CAD build for the part. Positions are in the model's coordinates, mm. Face numbers are marked on the shaded views. A direction names the side the tool comes from. Round coordinates to 2 decimals unless told otherwise and drop trailing zeros. Write each loop counter-clockwise with the first axis right and the second up, starting at its lowest first coordinate (ties: lowest second). Pieces come first, ordered by that corner, then holes. Notation, with made-up numbers: (51.25, -23) -> (67.25, -23) arc R13 cw to (67.25, -12) -> close; hole circle Ø9 at (62.5, -34). An arc over 180 degrees is marked (long way). Put each result on its own line as item: value. Start each with the question number.
1. Saw through at D-D on y = -15.5. List the corners of the cut face in (x, z), and give its area (3 significant figures).
2. Flat gauge pins, fed straight in: P1, Ø5, axis at x = -5.5, y = 14.5, coming from the +Z side; P2, Ø2, axis at x = -5.5, y = -16, coming from the +Z side; P3, Ø1.5, axis at x = -16, z = 7.5, coming from the -Y side; P4, Ø6, axis at x = -5.5, y = 15.5, coming from the +Z side. Where does each tip first touch, or does it go through?
3. Pull direction Y, two halves, no side cores. Call the marked faces 1, 2 and 3: pulls with the +Y half, pulls with the -Y half, needs draft (parallel to the pull), parting line crosses it, or undercut.
4. 3-axis set-ups, long thin cutter, end or side, ignore diameter. For the marked faces 4 and 5: which of +Z, -Z, +X, -X, +Y, -Y reach the whole face in a straight line?
5. Saw through at C-C on x = 10. List the corners of the cut face in (y, z), and give its area (3 significant figures).
6. Saw through at A-A on y = 0. List the corners of the cut face in (x, z), and give its area (3 significant figures).
7. Drill centre lines: line 1 (Y direction, x = 25.5, z = -0.95); line 2 (X direction, y = -15, z = -8.5); line 3 (Z direction, x = 33, y = 12). Where is each one in solid material? Low to high. Write a range as from..to.
8. Saw through at B-B on x = 25.5. List the corners of the cut face in (y, z), and give its area (3 significant figures).
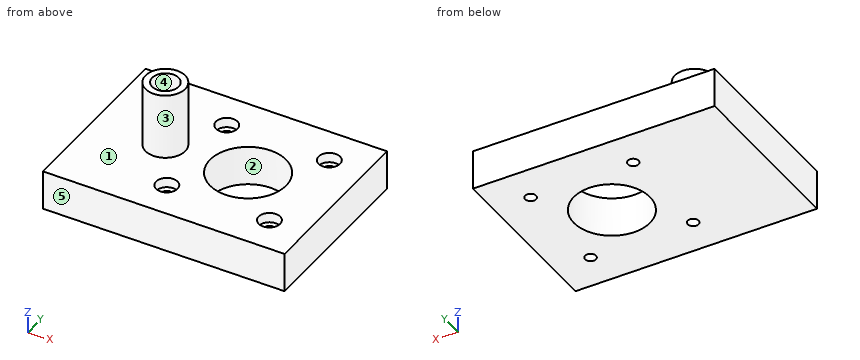
from build123d import *

# Parameters (mm, degrees)
F0_W           = 73
F0_H           = 53
F0_R           = 6
F0_R_2         = 11.5
F0_R_3         = 4
F1_DEPTH       = 12
F2_DEPTH       = 20
F3_D           = 3.3
F3_CBORE_D     = 6.5
F3_CBORE_DEPTH = 3


with BuildPart() as f1:
    # F0 (on Top) → F1 (new body)
    with BuildSketch(Plane.XY):
        Rectangle(F0_W, F0_H)
        with Locations((-15, 0)):
            Circle(F0_R, mode=Mode.SUBTRACT)
        with Locations((10, 0)):
            Circle(F0_R_2, mode=Mode.SUBTRACT)
        with Locations((-15, 0)):
            Circle(F0_R)
        with Locations((-15, 0)):
            Circle(F0_R_3, mode=Mode.SUBTRACT)
        with Locations((-15, 0)):
            Circle(F0_R_3)
    extrude(amount=-F1_DEPTH)

    # F0 (on Top) → F2 (join)
    with BuildSketch(Plane.XY):
        with Locations((-15, 0)):
            Circle(F0_R)
        with Locations((-15, 0)):
            Circle(F0_R_3, mode=Mode.SUBTRACT)
    extrude(amount=F2_DEPTH)

    # F3 (through all)
    with Locations(Plane.XY):
        with Locations((-5.5, 15.5), (25.5, 15.5), (25.5, -15.5), (-5.5, -15.5)):
            CounterBoreHole(F3_D / 2, F3_CBORE_D / 2, F3_CBORE_DEPTH)


solid = f1.part
Return value:
1. outline: (-36.5, -12) -> (-7.15, -12) -> (-7.15, -3) -> (-8.75, -3) -> (-8.75, 0) -> (-36.5, 0) -> close; (-3.85, -12) -> (23.85, -12) -> (23.85, -3) -> (22.25, -3) -> (22.25, 0) -> (-2.25, 0) -> (-2.25, -3) -> (-3.85, -3) -> close; (27.15, -12) -> (36.5, -12) -> (36.5, 0) -> (28.75, 0) -> (28.75, -3) -> (27.15, -3) -> close
1. area: 778 mm^2
2. P1: stops at z = 0
2. P2: passes through
2. P3: stops at y = -5.99
2. P4: stops at z = -3
3. face 1: needs draft
3. face 2: undercut
3. face 3: parting line crosses it
4. face 4: +Z
4. face 5: +Z, -Z, +X, -X, -Y
5. outline: (-26.5, -12) -> (-11.5, -12) -> (-11.5, 0) -> (-26.5, 0) -> close; (11.5, -12) -> (26.5, -12) -> (26.5, 0) -> (11.5, 0) -> close
5. area: 360 mm^2
6. outline: (-36.5, -12) -> (-1.5, -12) -> (-1.5, 0) -> (-9, 0) -> (-9, 20) -> (-11, 20) -> (-11, 0) -> (-19, 0) -> (-19, 20) -> (-21, 20) -> (-21, 0) -> (-36.5, 0) -> close; (21.5, -12) -> (36.5, -12) -> (36.5, 0) -> (21.5, 0) -> close
6. area: 680 mm^2
7. line 1: y = -26.5..-18.75, -12.25..12.25, 18.75..26.5
7. line 2: x = -36.5..-7.07, -3.93..23.93, 27.07..36.5
7. line 3: z = -12..0
8. outline: (-26.5, -12) -> (-17.15, -12) -> (-17.15, -3) -> (-18.75, -3) -> (-18.75, 0) -> (-26.5, 0) -> close; (-13.85, -12) -> (13.85, -12) -> (13.85, -3) -> (12.25, -3) -> (12.25, 0) -> (-12.25, 0) -> (-12.25, -3) -> (-13.85, -3) -> close; (17.15, -12) -> (26.5, -12) -> (26.5, 0) -> (18.75, 0) -> (18.75, -3) -> (17.15, -3) -> close
8. area: 538 mm^2
